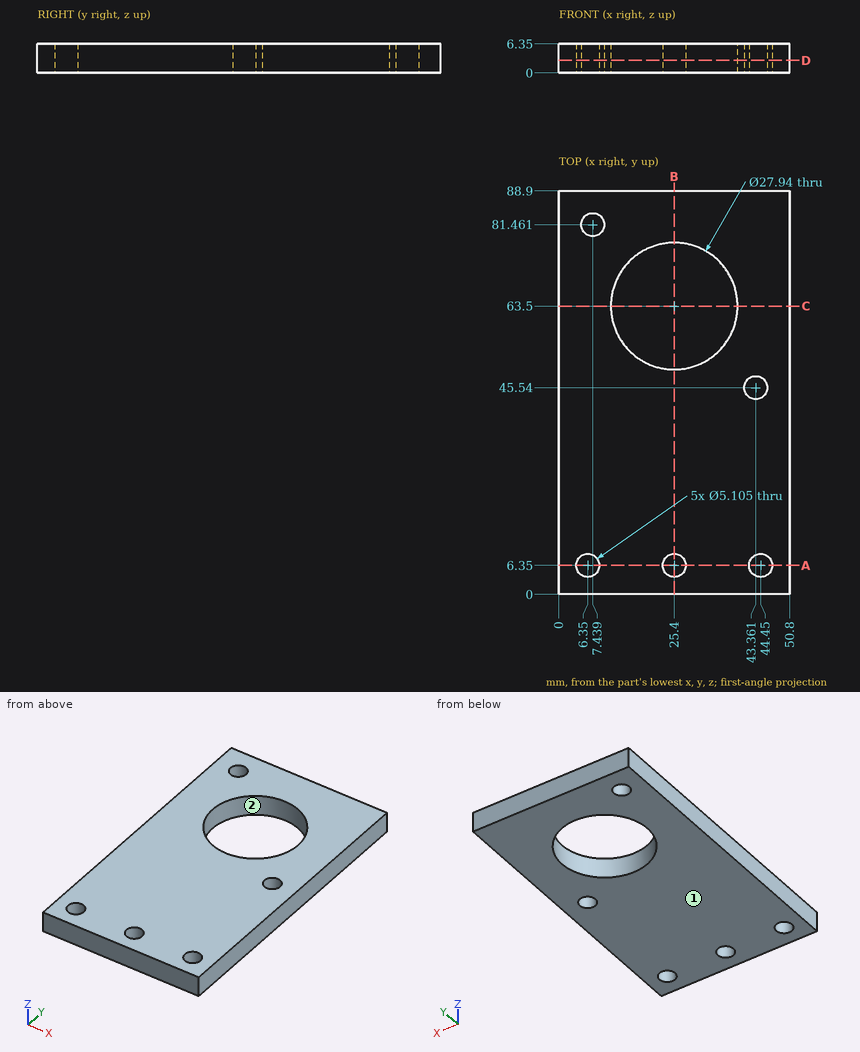
Part print with two shaded views. Sizes in mm from the minimum x, y, z corner. Round coordinates to 2 decimals unless told otherwise and drop trailing zeros. Order: outer loops, then holes, each group sorted by start corner. A loop starts at its lowest first (then second) coordinate and runs counter-clockwise, first axis right, second up. Notation, with made-up numbers: (32, -38.5) - (57, -38.5) arc R20 cw to (57, -15.5) - close; hole circle Ø7 at (29, 33.25). An arc over 180 degrees is marked (long way). Answer in a Markdown table with one row per item. Add a question column.
(1) Band-saw the part on C-C on y = 63.5. List the corners of the cut face in (x, z), and give its area (3 significant figures).
(2) Band-saw the part on A-A on y = 6.35. List the corners of the cut face in (x, z), and give its area (3 significant figures).
(3) Band-saw the part on B-B on x = 25.4. List the corners of the cut face in (y, z), and give its area (3 significant figures).
(4) Probe L1, parallel to X at y = 6.35, z = 4; L2, parallel to Y at x = 25.4, z = 4.5; L3, parallel to Y at x = 44.45, z = 3.5. List the from-to ranges inside material, lowest first. Write a range as [from, to].
(5) Band-saw the part on D-D on z = 2.75. Count the separate pieces of the cut face and the enclosed holes in it, and give its area (3 significant figures).
(6) Drop a flat-ended pin along its axis: pin 1 Ø3 at (x, y) = (43.36, 45.54) entering from +Z. Give the stop position or say it passes through.
(7) Mould opens along X. For the marked faces 1 and 2 say: +X half, -X half, draft (parallel to the pull), parting line (faces both ways), or undercut.
Data:
| question | item | result |
|---|---|---|
| 1 | outline | (0, 0) - (11.43, 0) - (11.43, 6.35) - (0, 6.35) - close; (39.37, 0) - (50.8, 0) - (50.8, 6.35) - (39.37, 6.35) - close |
| 1 | area | 145 mm^2 |
| 2 | outline | (0, 0) - (3.8, 0) - (3.8, 6.35) - (0, 6.35) - close; (8.9, 0) - (22.85, 0) - (22.85, 6.35) - (8.9, 6.35) - close; (27.95, 0) - (41.9, 0) - (41.9, 6.35) - (27.95, 6.35) - close; (47, 0) - (50.8, 0) - (50.8, 6.35) - (47, 6.35) - close |
| 2 | area | 225 mm^2 |
| 3 | outline | (0, 0) - (3.8, 0) - (3.8, 6.35) - (0, 6.35) - close; (8.9, 0) - (49.53, 0) - (49.53, 6.35) - (8.9, 6.35) - close; (77.47, 0) - (88.9, 0) - (88.9, 6.35) - (77.47, 6.35) - close |
| 3 | area | 355 mm^2 |
| 4 | L1 | x = [0, 3.8], [8.9, 22.85], [27.95, 41.9], [47, 50.8] |
| 4 | L2 | y = [0, 3.8], [8.9, 49.53], [77.47, 88.9] |
| 4 | L3 | y = [0, 3.8], [8.9, 43.23], [47.85, 88.9] |
| 5 | separate pieces | 1 |
| 5 | enclosed holes | 6 |
| 5 | area | 3,800 mm^2 |
| 6 | pin 1 | passes through |
| 7 | face 1 | draft |
| 7 | face 2 | undercut |
